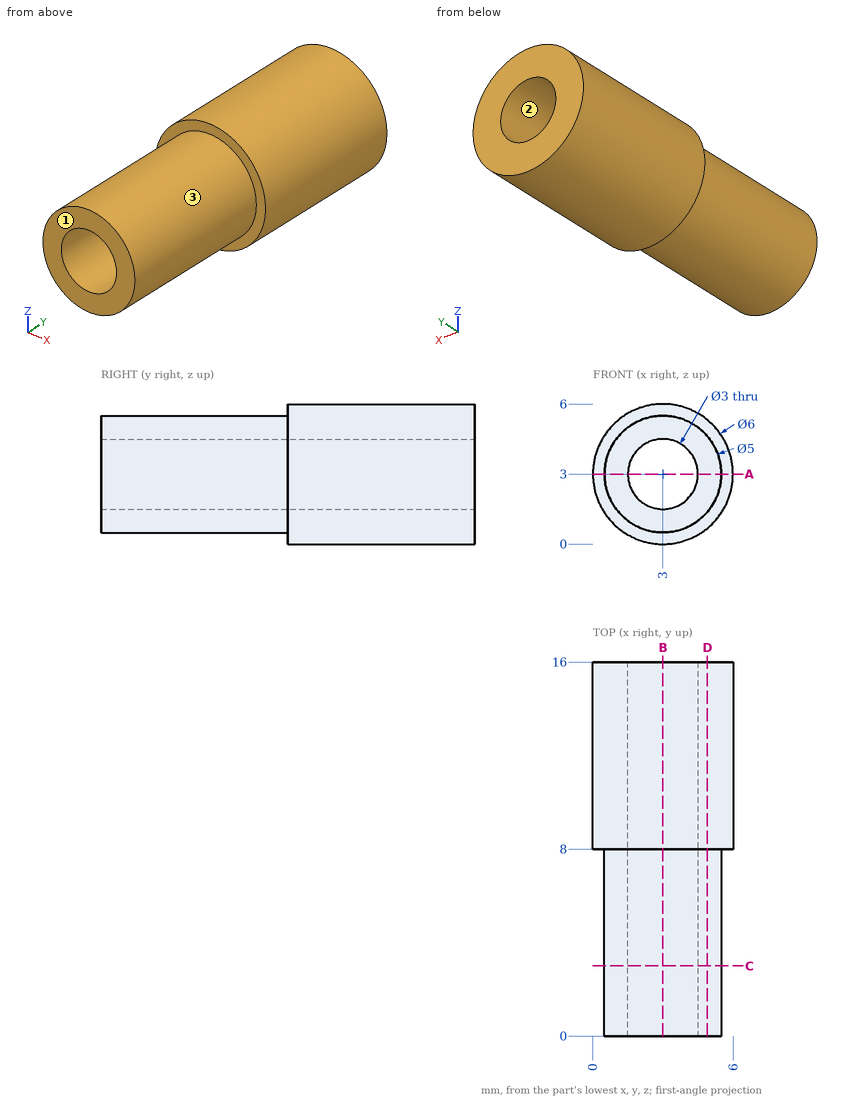
Geometry check sheet. Reference: drawing and pictorial views, mm from the part's lowest x, y, z. Round coordinates to 2 decimals unless told otherwise and drop trailing zeros. Loops run counter-clockwise (first coordinate to the right, second up) from the corner with the lowest first, then second, coordinate; pieces in that order, holes last. Notation, with made-up numbers: (-1, 71.25) - (53, 71.25) arc R13 cw to (53, 80.25) - close; hole circle Ø7 at (-36.5, -0.5). An arc over 180 degrees is marked (long way). Answer in a Markdown table with one row per item. Add a question column.
Q1. Section check C-C on y = 3. Enter the section's corners in (x, z).
Q2. Section check D-D on x = 4.9. Enter the section's corners in (y, z).
Q3. Section check B-B on x = 3. Enter the section's corners in (y, z), plus the area to 3 significant figures.
Q4. Section check A-A on z = 3. Enter the section's corners in (x, y), plus the area to 3 significant figures.
Q5. Release check for a two-part mould opening along X. For the marked faces 1, 2 and 3 record: pulls with the +X half, pulls with the -X half, needs draft (parallel to the pull), parting line crosses it, or undercut.
Q6. Material ranges on line 1 (Z direction, x = 3, y = 10.25); line 2 (Z direction, x = 3, y = 6.5); line 3 (Y direction, x = 2, z = 5.35), recorded low to high.
Q7. Gauge pin test, flat ends, axial feed: pin 1 (3 mm diameter, centred on x = 3.5, z = 3, fed in from -Y); pin 2 (2 mm diameter, centred on x = 2, y = 2, fed in from -Z). Record the tip position at first contact, or that the pin passes through.
Found:
| question | item | result |
|---|---|---|
| 1 | outline | circle Ø5 at (3, 3); hole circle Ø3 at (3, 3) |
| 2 | outline | (0, 1.38) - (8, 1.38) - (8, 0.68) - (16, 0.68) - (16, 5.32) - (8, 5.32) - (8, 4.62) - (0, 4.62) - close |
| 3 | outline | (0, 0.5) - (8, 0.5) - (8, 0) - (16, 0) - (16, 1.5) - (0, 1.5) - close; (0, 4.5) - (16, 4.5) - (16, 6) - (8, 6) - (8, 5.5) - (0, 5.5) - close |
| 3 | area | 40.0 mm² |
| 4 | outline | (0, 8) - (0.5, 8) - (0.5, 0) - (1.5, 0) - (1.5, 16) - (0, 16) - close; (4.5, 0) - (5.5, 0) - (5.5, 8) - (6, 8) - (6, 16) - (4.5, 16) - close |
| 4 | area | 40.0 mm² |
| 5 | face 1 | needs draft |
| 5 | face 2 | undercut |
| 5 | face 3 | parting line crosses it |
| 6 | line 1 | z = 0 to 1.5, 4.5 to 6 |
| 6 | line 2 | z = 0.5 to 1.5, 4.5 to 5.5 |
| 6 | line 3 | y = 8 to 16 |
| 7 | pin 1 | stops at y = 0 |
| 7 | pin 2 | stops at z = 0.5 |
